from build123d import *

# Parameters (mm, degrees)
F0_R     = 50
F0_R_2   = 10.5
F0_R_3   = 7.5
F1_DEPTH = 10
F2_DEPTH = 2


with BuildPart() as f1:
    # F0 (on Top) → F1 (new body)
    with BuildSketch(Plane.XY):
        Circle(F0_R)
        with Locations((0, -35)):
            Circle(F0_R_2, mode=Mode.SUBTRACT)
        with Locations((-35, 0)):
            Circle(F0_R_2, mode=Mode.SUBTRACT)
        Circle(F0_R_3, mode=Mode.SUBTRACT)
        with Locations((35, 0)):
            Circle(F0_R_2, mode=Mode.SUBTRACT)
        with Locations((0, 35)):
            Circle(F0_R_2, mode=Mode.SUBTRACT)
    extrude(amount=-F1_DEPTH)

    # F0 (on Top) → F2 (join)
    with BuildSketch(Plane.XY):
        Circle(F0_R)
        with Locations((0, -35)):
            Circle(F0_R_2, mode=Mode.SUBTRACT)
        with Locations((-35, 0)):
            Circle(F0_R_2, mode=Mode.SUBTRACT)
        Circle(F0_R_3, mode=Mode.SUBTRACT)
        with Locations((35, 0)):
            Circle(F0_R_2, mode=Mode.SUBTRACT)
        with Locations((0, 35)):
            Circle(F0_R_2, mode=Mode.SUBTRACT)
    extrude(amount=F2_DEPTH)


solid = f1.part
Read the model definition and answer for the solid it produces. Units are mm, in the model's axes. Round coordinates to 2 decimals unless told otherwise and drop trailing zeros. Order: outer loops, then holes, each group sorted by start corner. A loop starts at its lowest first (then second) coordinate and runs counter-clockwise, first axis right, second up. Notation, with made-up numbers: (51.25, 4.5) - (82.25, 4.5) arc R14 ccw to (82.25, 11.5) - close; hole circle Ø11 at (-14.5, -34.75). An arc over 180 degrees is marked (long way). Use one line per item in the form item = value. Start each with the question number.
(1) The part is cut by section C-C (x = -43.5). Give the vertices of the cut face in (y, z).
(2) The part is cut by section A-A (x = 0). Give the vertices of the cut face in (y, z).
(3) The part is cut by section D-D (y = -43). Give the vertices of the cut face in (x, z), then the cut area to 3 significant figures.
(4) Find the intervals of material crossed by line 1 along Y through (x, z) = (0, -6.75); line 2 along X through (y, z) = (-3.5, -6.5); line 3 along Y through (x, z) = (32, -7), in increasing order. Write a range as from..to.
(5) Flat-ended cylindrical pins translate along their axes: pin 1 Ø24 at (x, y) = (-35, 0) entering from +Z; pin 2 Ø19 at (x, y) = (0, 35) entering from -Z; pin 3 Ø1.5 at (x, z) = (2, -9) entering from +Y; pin 4 Ø1 at (x, z) = (-25.5, -6.5) entering from -Y. Find the tip coordinate at first contact, or state that the pin passes through.
Checked values:
q1.outline = (-24.65, -10) - (-6.16, -10) - (-6.16, 2) - (-24.65, 2) - close; (6.16, -10) - (24.65, -10) - (24.65, 2) - (6.16, 2) - close
q2.outline = (-50, -10) - (-45.5, -10) - (-45.5, 2) - (-50, 2) - close; (-24.5, -10) - (-7.5, -10) - (-7.5, 2) - (-24.5, 2) - close; (7.5, -10) - (24.5, -10) - (24.5, 2) - (7.5, 2) - close; (45.5, -10) - (50, -10) - (50, 2) - (45.5, 2) - close
q3.outline = (-25.51, -10) - (-6.8, -10) - (-6.8, 2) - (-25.51, 2) - close; (6.8, -10) - (25.51, -10) - (25.51, 2) - (6.8, 2) - close
q3.area = 449 mm^2
q4.line_1 = -50..-45.5, -24.5..-7.5, 7.5..24.5, 45.5..50
q4.line_2 = -49.88..-44.9, -25.1..-6.63, 6.63..25.1, 44.9..49.88
q4.line_3 = -38.42..-10.06, 10.06..38.42
q5.pin_1 = 2
q5.pin_2 = through
q5.pin_3 = 49.98
q5.pin_4 = -43.3
